Read the model definition and answer for the solid it produces. Units are mm, in the model's axes. Face numbers are marked on the shaded views. A direction names the side the tool comes from. Coordinates: 2 decimals unless noted, no trailing zeros. Loops run counter-clockwise (first coordinate to the right, second up) from the corner with the lowest first, then second, coordinate; pieces in that order, holes last. Notation, with made-up numbers: (81.5, -36) -> (102.5, -36) arc R18 ccw to (102.5, -13) -> close; hole circle Ø7 at (33.5, 7). An arc over 180 degrees is marked (long way). Answer as a JSON object with one key per item and string values. Group by question number.
Q1. Each of these flat-tipped pins is pushed along its axis until it touches: P1, Ø4, axis at x = 49.5, y = 15.5, coming from the -Z side; P2, Ø6, axis at y = 6.5, z = 11, coming from the -X side; P3, Ø7, axis at y = 17, z = 3.5, coming from the -X side. Where does it stop, or does it pass through?
Q2. The part is cut by section A-A on x = -49. Write down the section's boundary in (y, z) (3 decimals).
Q3. The part is cut by section C-C on y = 8.5. State how many separate pieces and enclosed holes the cut face has, and give its area (3 significant figures).
Q4. Straight lines are drawn through the part: line 1 along X through (y, z) = (15, 15) (3 decimals); line 2 along X through (y, z) = (4, 0); line 3 along Y through (x, z) = (-49, 16.65). For each, find the intervals that lie inside material, in ascending order. Write a range as [from, to].
Q5. The part is cut by section D-D on x = -26. Write down the section's boundary in (y, z), and give its area (3 significant figures).
Q6. The part is cut by section B-B on x = -4.5. Write down the section's boundary in (y, z), and give its area (3 significant figures).
Q7. For the marked faces 1, 2, 3 and 4, determine the directions among +Z, -Z, +X, -X, +Y, -Y from which every point of the face is accessible in a straight line to the end or side of a thin tool.
from build123d import *

# Parameters (mm, degrees)
F0_W     = 80
F0_H     = 28.5
F0_W_2   = 12
F0_H_2   = 4
F2_DEPTH = 30
F3_R     = 2
F4_R     = 2.5
F5_DEPTH = 17.25
F6_R     = 6
F8_DEPTH = 17.25
F4_R_2   = 4.125
F9_DEPTH = 16.25


# Not quite as in the source:
# - two fillets or chamfers of one size are made in one step


with BuildPart() as f2:
    # F0 (on Front) → F2 (new body)
    with BuildSketch(Plane.XZ):
        Polygon((43, 17.25), (-43, 17.25), (-43, 13.25), (-43, -17.25), (43, -17.25), (43, 13.25), align=None)
        Rectangle(F0_W, F0_H, mode=Mode.SUBTRACT)
        with Locations((49, 15.25)):
            Rectangle(F0_W_2, F0_H_2)
        with Locations((-49, 15.25)):
            Rectangle(F0_W_2, F0_H_2)
    extrude(amount=-F2_DEPTH)

    # F3
    f3_edges = [f2.edges().sort_by_distance(p)[0] for p in [
        (0, 0, -14.25),
        (0, 30, -14.25),
        (-43, 15, 13.25),
        (43, 15, 13.25),
        (55, 15, 13.25),
        (-55, 15, 13.25),
    ]]
    fillet(f3_edges, radius=F3_R)

    # F4 (on Top) → F5 (cut, through all)
    with BuildSketch(Plane.XY):
        with Locations((49, 15)):
            Circle(F4_R)
        with Locations((-49, 15)):
            Circle(F4_R)
    extrude(amount=F5_DEPTH, mode=Mode.SUBTRACT)

    # F6 (call 1 of 6: OpenCascade refuses the feature's edges together)
    f6_edges = [f2.edges().sort_by_distance(p)[0] for p in [
        (-40, 15, 14.25),
    ]]
    fillet(f6_edges, radius=F6_R)

    # F6#2 (call 2 of 6)
    f6_2_edges = [f2.edges().sort_by_distance(p)[0] for p in [
        (-40, 15, -14.25),
    ]]
    fillet(f6_2_edges, radius=F6_R)

    # F6#3 (call 3 of 6)
    f6_3_edges = [f2.edges().sort_by_distance(p)[0] for p in [
        (40, 15, 14.25),
    ]]
    fillet(f6_3_edges, radius=F6_R)

    # F6#4 (call 4 of 6)
    f6_4_edges = [f2.edges().sort_by_distance(p)[0] for p in [
        (40, 15, -14.25),
    ]]
    fillet(f6_4_edges, radius=F6_R)

    # F6#5 (call 5 of 6)
    f6_5_edges = [f2.edges().sort_by_distance(p)[0] for p in [
        (-43, 15, -17.25),
    ]]
    fillet(f6_5_edges, radius=F6_R)

    # F6#6 (call 6 of 6)
    f6_6_edges = [f2.edges().sort_by_distance(p)[0] for p in [
        (43, 15, -17.25),
    ]]
    fillet(f6_6_edges, radius=F6_R)

    # F1 (on Top) → F8 (cut, through all)
    with BuildSketch(Plane.XY):
        Polygon((38, 2), (38, 5.5), (34.5, 2), align=None)
        Polygon((38, 13.9852813742), (38, 22.4705627485), (17.5294372515, 2), (26.0147186258, 2), align=None)
        Polygon((9.0441558773, 2), (35.0441558773, 28), (26.558874503, 28), (0.558874503, 2), align=None)
        Polygon((-7.9264068712, 2), (18.0735931288, 28), (9.5883117546, 28), (-16.4116882454, 2), align=None)
        Polygon((-24.8969696197, 2), (1.1030303803, 28), (-7.3822509939, 28), (-33.3822509939, 2), align=None)
        Polygon((-38, 5.8675323681), (-15.8675323681, 28), (-24.3528137424, 28), (-38, 14.3528137424), align=None)
        Polygon((-38, 22.8380951166), (-32.8380951166, 28), (-38, 28), align=None)
    extrude(amount=-F8_DEPTH, mode=Mode.SUBTRACT)

    # F4 (on Top) → F9 (cut)
    with BuildSketch(Plane.XY):
        with Locations((-49, 15)):
            Circle(F4_R_2)
        with Locations((-49, 15)):
            Circle(F4_R, mode=Mode.SUBTRACT)
        with Locations((49, 15)):
            Circle(F4_R_2)
        with Locations((49, 15)):
            Circle(F4_R, mode=Mode.SUBTRACT)
    extrude(amount=F9_DEPTH, mode=Mode.SUBTRACT)


solid = f2.part
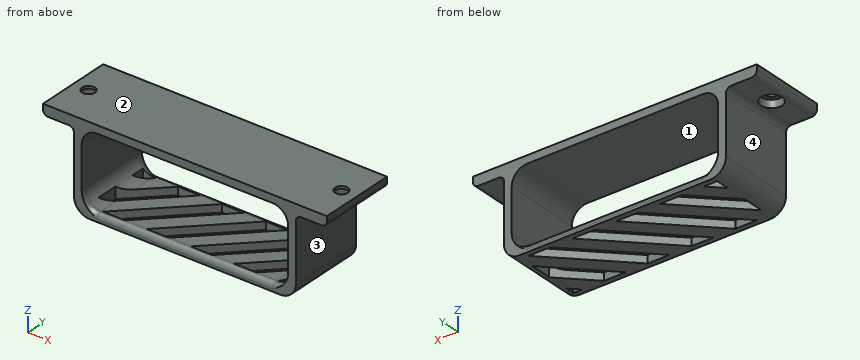
Final values:
{
 "1": {"P1": "stops at z = 16.25", "P2": "stops at x = -54.56", "P3": "stops at x = -43"},
 "2": {"outline": "(0, 13.25) -> (10.875, 13.25) -> (10.875, 16.25) -> (12.5, 16.25) -> (12.5, 17.25) -> (0, 17.25) -> close; (17.5, 16.25) -> (19.125, 16.25) -> (19.125, 13.25) -> (30, 13.25) -> (30, 17.25) -> (17.5, 17.25) -> close"},
 "3": {"separate pieces": "5", "enclosed holes": "0", "area": "687 mm2"},
 "4": {"line 1": "x = [-54.984, -53.125], [-44.875, 44.875], [53.125, 54.984]", "line 2": "x = [-43, -40], [40, 43]", "line 3": "y = [0, 12.5], [17.5, 30]"},
 "5": {"outline": "(0, -17.25) -> (2, -17.25) -> (2, -14.25) arc R2 ccw to (0, -16.25) -> close; (0, 14.25) -> (30, 14.25) -> (30, 17.25) -> (0, 17.25) -> close; (9.38, -17.25) -> (17.87, -17.25) -> (17.87, -14.25) -> (9.38, -14.25) -> close; (26.35, -17.25) -> (30, -17.25) -> (30, -16.25) arc R2 ccw to (28, -14.25) -> (26.35, -14.25) -> close", "area": "131 mm2"},
 "6": {"outline": "(0, -17.25) -> (5.43, -17.25) -> (5.43, -14.25) -> (2, -14.25) arc R2 ccw to (0, -16.25) -> close; (0, 14.25) -> (30, 14.25) -> (30, 17.25) -> (0, 17.25) -> close; (13.91, -17.25) -> (22.4, -17.25) -> (22.4, -14.25) -> (13.91, -14.25) -> close; (28, -17.25) -> (30, -17.25) -> (30, -16.25) arc R2 ccw to (28, -14.25) -> close", "area": "136 mm2"},
 "7": {"face 1": "+Y, -Y", "face 2": "+Z, +X, -X, +Y, -Y", "face 3": "-Z, +X, +Y, -Y", "face 4": "-Z, -X, +Y, -Y"}
}
